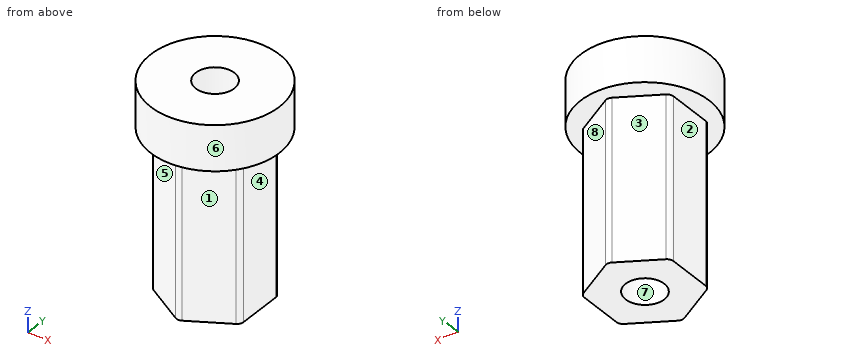
from build123d import *

# Parameters (mm, degrees)
CUT_EXTRUDE1_DEPTH = 25
FILLET1_R          = 1


with BuildPart() as part:
    # Sketch2 → Revolve1 (revolve)
    with BuildSketch(Plane(origin=(0, 0, 0), x_dir=(0, 0, -1), z_dir=(1, 0, 0))):
        Polygon((-7, 3), (25, 3), (25, 8), (0, 8), (0, 10), (-7, 10), align=None)
    revolve(axis=Axis((0, 0, 0), (0, 0, -1)))

    # Sketch3 → Cut-Extrude1 (cut)
    with BuildSketch(Plane(origin=(0, 0, -25), x_dir=(-1, 0, 0), z_dir=(0, 0, -1))):
        with BuildLine():
            ThreePointArc((0, 8), (-4, 6.92820323), (-6.92820323, 4))
            Line((-6.92820323, 4), (0, 8))
        make_face()
        with BuildLine():
            ThreePointArc((-6.92820323, 4), (-8, 0), (-6.92820323, -4))
            Line((-6.92820323, -4), (-6.92820323, 4))
        make_face()
        with BuildLine():
            ThreePointArc((-6.92820323, -4), (-4, -6.92820323), (0, -8))
            Line((0, -8), (-6.92820323, -4))
        make_face()
        with BuildLine():
            Line((6.92820323, -4), (0, -8))
            ThreePointArc((0, -8), (4, -6.92820323), (6.92820323, -4))
        make_face()
        with BuildLine():
            Line((6.92820323, 4), (6.92820323, -4))
            ThreePointArc((6.92820323, -4), (7.72740661, -2.070552361), (8, 0))
            ThreePointArc((8, 0), (7.72740661, 2.070552361), (6.92820323, 4))
        make_face()
        with BuildLine():
            Line((0, 8), (6.92820323, 4))
            ThreePointArc((6.92820323, 4), (4, 6.92820323), (0, 8))
        make_face()
    extrude(amount=-CUT_EXTRUDE1_DEPTH, mode=Mode.SUBTRACT)

    # Fillet1
    fillet1_edges = [part.edges().sort_by_distance(p)[0] for p in [
        (0, 8, -12.5),
        (6.92820323, 4, -12.5),
        (6.92820323, -4, -12.5),
        (0, -8, -12.5),
        (-6.92820323, -4, -12.5),
        (-6.92820323, 4, -12.5),
    ]]
    fillet(fillet1_edges, radius=FILLET1_R)


solid = part.part
Read the model definition and answer for the solid it produces. Units are mm, in the model's axes. Face numbers are marked on the shaded views. A direction names the side the tool comes from. Round coordinates to 2 decimals unless told otherwise and drop trailing zeros. Write each loop counter-clockwise with the first axis right and the second up, starting at its lowest first coordinate (ties: lowest second). Pieces come first, ordered by that corner, then holes. Notation, with made-up numbers: M 14,42.25 L 52,42.25 A20 ccw 52,80.25 Z; hole C 5,85 d7. An arc over 180 degrees is marked long. Use a Markdown table: item, result.
1) The part is cut by section D-D (y = 6). Write down the section's boundary in (x, z).
Answers follow:
| item | result |
|---|---|
| outline | M -8,0 L -3.46,0 L -3.46,-25 L 3.46,-25 L 3.46,0 L 8,0 L 8,7 L -8,7 Z |
2) For a pull along X with two mould halves and no side action, classify the marked faces 6, 7 and 8 as pulls with the +X half, pulls with the -X half, needs draft (parallel to the pull), parting line crosses it, or undercut.
Answers follow:
| item | result |
|---|---|
| face 6 | parting line crosses it |
| face 7 | undercut |
| face 8 | pulls with the +X half |
3) The part is cut by section B-B (x = 0). Write down the section's boundary in (y, z), plus the area to 3 significant figures.
Answers follow:
| item | result |
|---|---|
| outline | M -10,0 L -7.85,0 L -7.85,-25 L -3,-25 L -3,7 L -10,7 Z; M 3,-25 L 7.85,-25 L 7.85,0 L 10,0 L 10,7 L 3,7 Z |
| area | 340 mm2 |
4) A tool of negligible diameter and unlimited length cuts with its end or side. For the marked faces 1, 2, 3, 4 and 5, from which of +Z, -Z, +X, -X, +Y, -Y can it reach the whole face along a straight path? Write none if from no direction.
Answers follow:
| item | result |
|---|---|
| face 1 | -Z, +X, -Y |
| face 2 | -Z, -X, +Y, -Y |
| face 3 | -Z, -X, +Y |
| face 4 | -Z, +X, +Y, -Y |
| face 5 | -Z, -X, -Y |
5) Flat-ended cylindrical pins translate along their axes: pin 1 (2 mm diameter, centred on x = 4.5, z = -8.5, fed in from -Y); pin 2 (7.5 mm diameter, centred on y = 0, z = -6.5, fed in from +X); pin 3 (6 mm diameter, centred on y = 3.5, z = 2, fed in from +X). Find the tip coordinate at first contact, or state that the pin passes through.
Answers follow:
| item | result |
|---|---|
| pin 1 | stops at y = -5.98 |
| pin 2 | stops at x = 6.93 |
| pin 3 | stops at x = 9.99 |
6) Straight lines are drawn through the part: line 1 along X through (y, z) = (0, 1); line 2 along X through (y, z) = (0, -5.5); line 3 along Z through (x, y) = (8.75, 3). For each, find the intervals that lie inside material, in ascending order. Write a range as [from, to].
Answers follow:
| item | result |
|---|---|
| line 1 | x = [-10, -3], [3, 10] |
| line 2 | x = [-6.93, -3], [3, 6.93] |
| line 3 | z = [0, 7] |
7) The part is cut by section C-C (z = -4). Write down the section's boundary in (x, y), plus the area to 3 significant figures.
Answers follow:
| item | result |
|---|---|
| outline | M -6.93,-3.42 A1 ccw -6.43,-4.29 L -0.5,-7.71 A1 ccw 0.5,-7.71 L 6.43,-4.29 A1 ccw 6.93,-3.42 L 6.93,3.42 A1 ccw 6.43,4.29 L 0.5,7.71 A1 ccw -0.5,7.71 L -6.43,4.29 A1 ccw -6.93,3.42 Z; hole C 0,0 d6 |
| area | 138 mm2 |
8) The part is cut by section A-A (y = 0). Write down the section's boundary in (x, z), plus the area to 3 significant figures.
Answers follow:
| item | result |
|---|---|
| outline | M -10,0 L -6.93,0 L -6.93,-25 L -3,-25 L -3,7 L -10,7 Z; M 3,-25 L 6.93,-25 L 6.93,0 L 10,0 L 10,7 L 3,7 Z |
| area | 294 mm2 |
